Here's how the part is built. I have some questions about the finished solid (model axes, mm). A direction names the side the tool comes from. Round coordinates to 2 decimals unless told otherwise and drop trailing zeros. Write each loop counter-clockwise with the first axis right and the second up, starting at its lowest first coordinate (ties: lowest second). Pieces come first, ordered by that corner, then holes. Notation, with made-up numbers: M 69.5,24 L 81.5,24 A24 cw 81.5,50 Z; hole C 11,59.5 d5. An arc over 180 degrees is marked long. Use one line per item in the form item = value. Start each with the question number.
Q1. I want a section at A-A on y = 0. List the corners of the cut face in (x, z) for me (3 decimals).
Q2. We'd pull the mould along Y, two halves only. Please class faces 3 (the face through (-9.727, -0.088, 1.521)), 4 (the face through (3, -3, 3)), 5 (the face through (-1.72, -7.76, -4.93)): +Y half, -Y half, draft (parallel to the pull), parting line (faces both ways), or undercut.
Q3. I'm going to push flat-ended pins straight in: pin 1 Ø5 at (y, z) = (5.5, -4) entering from -X; pin 2 Ø3 at (x, z) = (-6, -3.5) entering from -Y; pin 3 Ø4 at (y, z) = (-8, -6) entering from +X. Where does each tip first touch, or does it pass through?
Q4. For faces 1 (the face through (0.088, -9.727, 1.521)), 2 (the face through (-7, -7, 0)), which set-ups out of +Z, -Z, +X, -X, +Y, -Y let a thin tool reach every point of the face, with its end or its side?
Q5. I need wall thicknesses on line 1 along Y through (x, z) = (1, 1.25); line 2 along Y through (x, z) = (0, -5.75); line 3 along Z through (x, y) = (-10, -7). Which ranges of each line are inside material? Lowest first, please. Write a range as from..to.
Q6. I want a section at D-D on z = 1.25. List the corners of the cut face in (x, y) for me (3 decimals).
Q7. I want a section at C-C on x = -12. List the corners of the cut face in (y, z) for me.
```python
from build123d import *

# Parameters (mm, degrees)
SKETCH009_R           = 2
POCKET001_DEPTH       = 101.455907
POCKET001_DEPTH_BACK  = 94.455907
POLARPATTERN001_COUNT = 4


with BuildPart() as part:
    # Sketch008 → Revolution005 (revolve)
    with BuildSketch(Plane.XZ):
        Polygon((4.05, 3), (4.05, -10), (7.95, -10), (7.95, 0), (15.5, 0), (15.5, 3), align=None)
    revolve(axis=Axis((0, 0, 0), (0, 0, 1)))

    # Sketch009 → Pocket001 (cut, two sides)
    with BuildSketch(Plane.XY) as pocket001_sk:
        with Locations((11.725, 0)):
            Circle(SKETCH009_R)
    pocket001 = extrude(amount=-POCKET001_DEPTH, mode=Mode.SUBTRACT) + extrude(pocket001_sk.sketch, amount=POCKET001_DEPTH_BACK, mode=Mode.SUBTRACT)

    # PolarPattern001: Pocket001 ×4 about axis
    polarpattern001_axis = Axis((0, 0, 0), (0, 0, 1))
    for i in range(1, POLARPATTERN001_COUNT):
        add(pocket001.rotate(polarpattern001_axis, i * 360 / POLARPATTERN001_COUNT), mode=Mode.SUBTRACT)


solid = part.part
```
Reported:
q1.outline = M -15.5,0 L -13.725,0 L -13.725,3 L -15.5,3 Z; M -9.725,0 L -7.95,0 L -7.95,-10 L -4.05,-10 L -4.05,3 L -9.725,3 Z; M 4.05,-10 L 7.95,-10 L 7.95,0 L 9.725,0 L 9.725,3 L 4.05,3 Z; M 13.725,0 L 15.5,0 L 15.5,3 L 13.725,3 Z
q2.face_3 = undercut
q2.face_4 = draft
q2.face_5 = parting line
q3.pin_1 = -7.36
q3.pin_2 = -6.55
q3.pin_3 = 5.22
q4.face_1 = +Z, -Z
q4.face_2 = -Z
q5.line_1 = -15.47..-13.46, -9.99..-3.92, 3.92..9.99, 13.46..15.47
q5.line_2 = -7.95..-4.05, 4.05..7.95
q5.line_3 = 0..3
q6.outline = C 0,0 d31; hole C -11.725,0 d4; hole C 0,0 d8.1; hole C 0,-11.725 d4; hole C 0,11.725 d4; hole C 11.725,0 d4
q7.outline = M -9.81,0 L -1.98,0 L -1.98,3 L -9.81,3 Z; M 1.98,0 L 9.81,0 L 9.81,3 L 1.98,3 Z
